Design review of the part built by this model. Coordinates are the model's own, in mm. Face numbers are marked on the shaded views. A direction names the side the tool comes from. Give positions to 0.01 mm unless a question says otherwise; leave off trailing zeros. Order: outer loops, then holes, each group sorted by start corner. A loop starts at its lowest first (then second) coordinate and runs counter-clockwise, first axis right, second up.
Autodesk Fusion 360 part; units mm, degrees
sketch "Skizze1" plane through (0, 0, 0) normal (0, 1, 0) x (1, 0, 0)
  line L0 (0, 0) -> (0, -15)
  line L1 (0, -15) -> (15, -15)
  line L2 (15, -15) -> (15, 0)
  line L3 (15, 0) -> (0, 0)
  line L4 (15, 0) -> (17.5, 0)
  line L5 (17.5, 0) -> (17.5, -15)
  line L6 (17.5, -15) -> (15, -15)
  dimension "d1" = 15
  dimension "d2" = 15
  dimension "d3" = 2.5
sketch "Skizze2" plane through (0, 13, 0) normal (0, 1, 0) x (-1, 0, 0)
sketch "Skizze3" plane through (0, 0, 0) normal (0, 1, 0) x (1, 0, 0)
  line L0 (0, 0) -> (0, -15)
  line L1 (0, -15) -> (0, 0)
  circle A0 centre (0, 0) radius 15
  line L2 (0, 0) -> (-10.3643, -10.8435)
extrude "Extrusion2" add sketch "Skizze3" along normal blind 9 contours L0 L1 A0 L2 picked at (-1.8916, -9.7989)
sketch "Skizze4" plane through (0, 0, 0) normal (-0.7229, 0, -0.691) x (-0.691, 0, 0.7229)
  line L0 (0, 0) -> (15, 0)
  line L1 (15, 0) -> (15, 9)
  line L2 (15, 9) -> (0, 9)
  line L3 (0, 9) -> (0, 0)
  circle A0 centre (2.6906, 2.7068) radius 0.759
  circle A1 centre (3.9712, 6.7561) radius 1.6237
  circle A2 centre (11.6545, 6.7561) radius 1.1059
  circle A3 centre (7.6744, 3.9181) radius 0.5299
  circle A4 centre (7.6744, 6.7561) radius 0.6239
  circle A5 centre (9, 1.5) radius 0.8703
  circle A6 centre (11.7237, 4.0566) radius 1.4228
extrude "Extrusion3" cut sketch "Skizze4" against normal blind 1 contours A0 | A1 | A2 | A3 | A4 | A5 | A6
sketch "Skizze5" plane through (0, 9, 0) normal (0, 1, 0) x (-1, 0, 0)
  line L0 (0, 0) -> (10.3643, 10.8435)
  arc A0 (10.3643, 10.8435) -> (0, 15) centre (0, 0) ccw
  line L1 (0, 15) -> (0, 0)
  circle A1 centre (2.6465, 11.993) radius 1.5376
  circle A2 centre (2.6465, 6.4536) radius 1.1912
  circle A3 centre (6.1213, 10.6395) radius 0.8189
  circle A4 centre (5.1094, 8.4518) radius 0.4
extrude "Extrusion4" cut sketch "Skizze5" against normal blind 1 contours A1 | A2 | A3 | A4
sketch "Skizze6" plane through (0, 0, 0) normal (1, 0, 0) x (0, 0, -1)
  line L0 (-15, 0) -> (0, 0)
  line L1 (0, 0) -> (0, 9)
  line L2 (0, 9) -> (-15, 9)
  line L3 (-15, 9) -> (-15, 0)
  circle A0 centre (-11.6448, 6.5689) radius 1.5047
  circle A1 centre (-10.1749, 3.2155) radius 0.7721
  circle A2 centre (-4.3869, 6.3622) radius 0.7676
  circle A3 centre (-5.9028, 3.2155) radius 0.5958
  circle A4 centre (-2.4117, 3.9046) radius 1.2257
  circle A5 centre (-7.924, 5.5353) radius 0.9866
  circle A6 centre (-6.7297, 2.2968) radius 0.8791
extrude "Extrusion5" cut sketch "Skizze6" against normal blind 1 contours A0 | A1 | A2 | A3 A6 | A3 A6 | A3 A6 | A4 | A5
sketch "Skizze7" plane through (0, 0, 0) normal (0, 0, 1) x (1, 0, 0)
  circle A0 centre (-7.7636, 6.803) radius 1.5064
  circle A1 centre (-2.9408, 5.4698) radius 1.0472
  circle A2 centre (-5.8227, 2.6859) radius 1.6102
ref_plane "Arbeitsebene1" through (-7.7636, 6.803, 16) normal (0, 0, 1) x (1, 0, 0)
sketch "Skizze8" plane through (0, 0, 16) normal (0, 0, 1) x (1, 0, 0)
  circle A0 centre (-7.7283, 6.7967) radius 1.4872
  circle A1 centre (-5.8039, 2.6728) radius 1.6738
  circle A2 centre (-2.8714, 5.4221) radius 1.1553
extrude "Extrusion6" cut sketch "Skizze8" against normal blind 2
extrude "Extrusion7" cut sketch "Skizze8" against normal blind 4 contours A0
sketch "Skizze9" plane through (0, 0, 0) normal (0, -1, 0) x (1, 0, 0)
  line L0 (-10.3643, 10.8435) -> (0, 0)
  line L1 (0, 0) -> (0, 15)
  arc A0 (0, 15) -> (-10.3643, 10.8435) centre (0, 0) ccw
  line L2 (0, 0) -> (-5.5833, 13.9222)
  circle A1 centre (-4.3092, 10.7452) radius 1.85
  dimension "d19" = 3.7
extrude "Extrusion8" cut sketch "Skizze9" against normal blind 7 contours L2 A1 | L2 A1
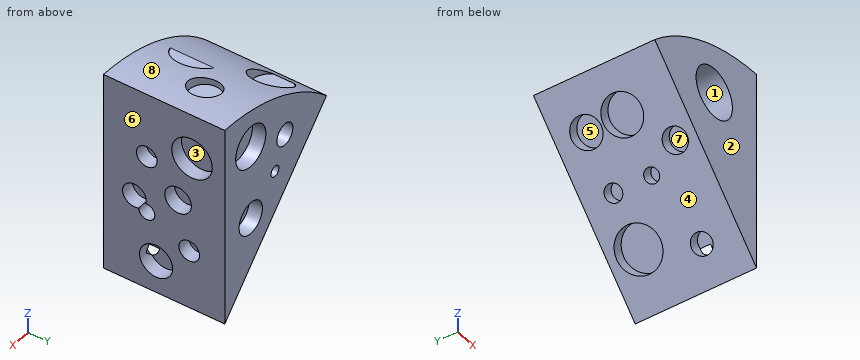
1. For pin 1 (1.8 mm diameter, centred on x = -5, z = 11.5, fed in from -Y); pin 2 (3 mm diameter, centred on y = 7.5, z = 3, fed in from -X); pin 3 (2 mm diameter, centred on x = -9, y = 5, fed in from +Z); pin 4 (3 mm diameter, centred on x = -8, y = 7.5, fed in from +Z), all flat-tipped, find the tip position at first contact; note any pin that passes through.
Recorded:
pin 1: stops at y = 0
pin 2: stops at x = -4.3
pin 3: stops at z = 12.69
pin 4: stops at z = 13.52
2. Take a section at A-A (z = 1). State the section outline as (x, y) points.
Recorded:
outline: (-0.96, 0) - (0, 0) - (0, 9) - (-0.96, 9) - close
3. Draft analysis for pull direction Z (two halves, no side actions). For the marked faces 6, 7 and 8, state which applies: pulls with the +Z half, pulls with the -Z half, needs draft (parallel to the pull), parting line crosses it, or undercut.
Recorded:
face 6: needs draft
face 7: undercut
face 8: pulls with the +Z half
4. For line 1 along Y through (x, z) = (-1.5, 12.5); line 2 along X through (y, z) = (8.75, 12.25); line 3 along Y through (x, z) = (-5.5, 6.5), list the stretches that pass through material, from the lowest coordinate up.
Recorded:
line 1: y = 0 to 8
line 2: x = -8.66 to -4.16, -1.13 to 0
line 3: y = 0 to 0.79, 2.21 to 9
5. Machinability: for the marked faces 1, 2, 3, 4 and 5, which of the approach directions +Z, -Z, +X, -X, +Y, -Y give a long, thin tool a straight path to every point of the face, cutting with its end or side? Answer none if there is none.
Recorded:
face 1: -Y
face 2: +Z, -Z, +X, -X, -Y
face 3: +X
face 4: -Z, -X, +Y, -Y
face 5: none
